from build123d import *

# Parameters (mm, degrees)
SKETCH1_R           = 4
SKETCH1_R_2         = 22.5
SKETCH1_R_3         = 1.5
SKETCH1_R_4         = 2
SKETCH1_W           = 13.5
SKETCH1_H           = 6.5
BOSS_EXTRUDE1_DEPTH = 5


with BuildPart() as part:
    # Sketch1 → Boss-Extrude1 (new body)
    with BuildSketch(Plane.XY):
        with BuildLine():
            Line((61, -35), (-61, -35))
            ThreePointArc((-61, -35), (-96, 0), (-61, 35))
            Line((-61, 35), (61, 35))
            ThreePointArc((61, 35), (96, 0), (61, -35))
        make_face()
        with Locations((61, 0)):
            Circle(SKETCH1_R, mode=Mode.SUBTRACT)
        with Locations((-61, 0)):
            Circle(SKETCH1_R_2, mode=Mode.SUBTRACT)
        with Locations((-61, -29)):
            Circle(SKETCH1_R_3, mode=Mode.SUBTRACT)
        with Locations((-61, 29)):
            Circle(SKETCH1_R_3, mode=Mode.SUBTRACT)
        with Locations((61, 29)):
            Circle(SKETCH1_R_3, mode=Mode.SUBTRACT)
        with Locations((61, -29)):
            Circle(SKETCH1_R_3, mode=Mode.SUBTRACT)
        with Locations((0, 29)):
            Circle(SKETCH1_R_3, mode=Mode.SUBTRACT)
        with Locations((-90, 0)):
            Circle(SKETCH1_R_3, mode=Mode.SUBTRACT)
        with Locations((-32, 0)):
            Circle(SKETCH1_R_3, mode=Mode.SUBTRACT)
        with Locations((90, 0)):
            Circle(SKETCH1_R_3, mode=Mode.SUBTRACT)
        with Locations((32, 0)):
            Circle(SKETCH1_R_3, mode=Mode.SUBTRACT)
        with Locations((61, 12)):
            Circle(SKETCH1_R_4, mode=Mode.SUBTRACT)
        with Locations((61, -12)):
            Circle(SKETCH1_R_4, mode=Mode.SUBTRACT)
        with Locations((49, 0)):
            Circle(SKETCH1_R_4, mode=Mode.SUBTRACT)
        with Locations((73, 0)):
            Circle(SKETCH1_R_4, mode=Mode.SUBTRACT)
        with Locations((10.75, -6.75)):
            Circle(SKETCH1_R_4, mode=Mode.SUBTRACT)
        with Locations((17.75, -6.75)):
            Circle(SKETCH1_R_4, mode=Mode.SUBTRACT)
        with Locations((-23.054905042, 20.964824554)):
            Circle(SKETCH1_R_4, mode=Mode.SUBTRACT)
        with Locations((-29.435230641, 18.085337577)):
            Circle(SKETCH1_R_4, mode=Mode.SUBTRACT)
        with Locations((0, -29)):
            Circle(SKETCH1_R_3, mode=Mode.SUBTRACT)
        with Locations((14.25, 0)):
            Rectangle(SKETCH1_W, SKETCH1_H, mode=Mode.SUBTRACT)
        Polygon((-30.95778118, 13.55827011), (-28.283971844, 7.633682054), (-15.979058189, 13.186978367), (-18.652867525, 19.111566423), align=None, mode=Mode.SUBTRACT)
    extrude(amount=BOSS_EXTRUDE1_DEPTH)


solid = part.part
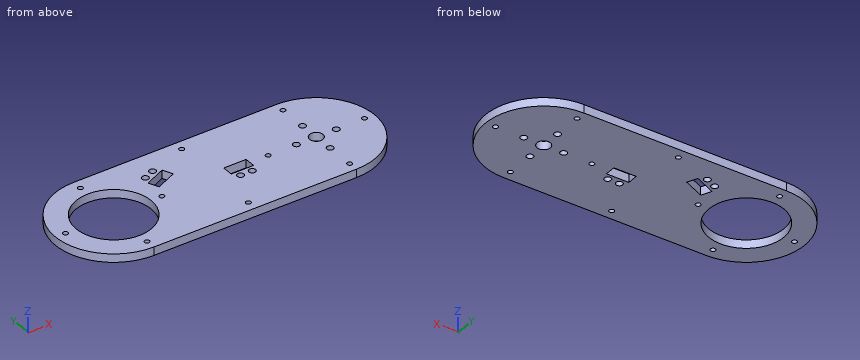
Build history of the part. All positions in model axes, mm. Give positions to 0.01 mm unless a question says otherwise; leave off trailing zeros. Loops run counter-clockwise (first coordinate to the right, second up) from the corner with the lowest first, then second, coordinate; pieces in that order, holes last. Notation, with made-up numbers: (21.25, 74) -> (61.25, 74) arc R20 cw to (61.25, 88) -> close; hole circle Ø7 at (-30.75, 26.5). An arc over 180 degrees is marked (long way). Answer in a Markdown table with one row per item.
Item 1: Slice it at B-B on y = -12. Write the cut outline in (x, z).
Findings below:
| item | result |
|---|---|
| outline | (-93.88, 0) -> (-80.03, 0) -> (-80.03, 5) -> (-93.88, 5) -> close; (-41.97, 0) -> (59, 0) -> (59, 5) -> (-41.97, 5) -> close; (63, 0) -> (93.88, 0) -> (93.88, 5) -> (63, 5) -> close |
Item 2: Slice it at C-C on x = -81.5. Write the cut outline in (y, z).
Findings below:
| item | result |
|---|---|
| outline | (-28.37, 0) -> (-9.27, 0) -> (-9.27, 5) -> (-28.37, 5) -> close; (9.27, 0) -> (28.37, 0) -> (28.37, 5) -> (9.27, 5) -> close |
Item 3: Flat gauge pins, fed straight in: P1, Ø2.5, axis at x = 0, y = 29, coming from the -Z side; P2, Ø1.5, axis at y = -24.5, z = 1.5, coming from the +X side; P3, Ø2.5, axis at y = -0.5, z = 2, coming from the -X side. Where does each tip first touch, or does it go through?
Findings below:
| item | result |
|---|---|
| P1 | passes through |
| P2 | stops at x = 86.71 |
| P3 | stops at x = -96 |
Item 4: Slice it at D-D on z = 1.7. Give the number of separate pieces and of enclosed holes in the cut face, plus the area to 3 significant figures.
Findings below:
| item | result |
|---|---|
| separate pieces | 1 |
| enclosed holes | 22 |
| area | 10,400 mm² |
Item 5: Probe line 1 along Y through (x, z) = (-61, 2.4); line 2 along Y through (x, z) = (-32, 1.25); line 3 along X through (y, z) = (18, 0.3). List the from-to ranges inside material, lowest first. Write a range as [from, to].
Findings below:
| item | result |
|---|---|
| line 1 | y = [-35, -30.5], [-27.5, -22.5], [22.5, 27.5], [30.5, 35] |
| line 2 | y = [-35, -1.5], [1.5, 35] |
| line 3 | x = [-91.02, -74.5], [-47.5, -31.43], [-27.44, -21.12], [-18.15, 91.02] |
Item 6: Slice it at A-A on x = 17.75. Write the cut outline in (y, z).
Findings below:
| item | result |
|---|---|
| outline | (-35, 0) -> (-8.75, 0) -> (-8.75, 5) -> (-35, 5) -> close; (-4.75, 0) -> (-3.25, 0) -> (-3.25, 5) -> (-4.75, 5) -> close; (3.25, 0) -> (35, 0) -> (35, 5) -> (3.25, 5) -> close |
